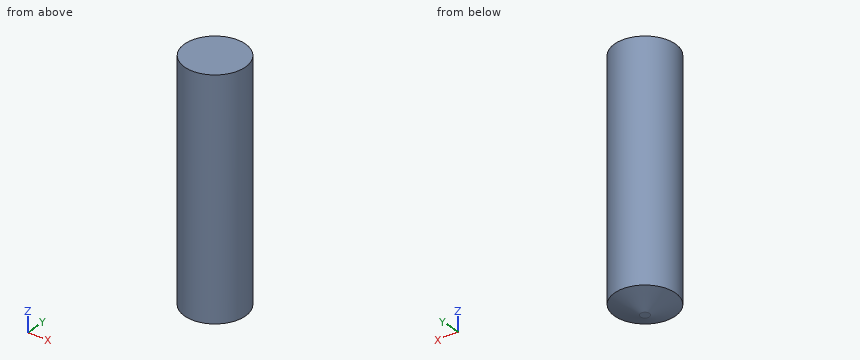
from build123d import *

# Parameters (mm, degrees)
CYLINDER_R     = 2.5
CYLINDER_DEPTH = 20


with BuildPart() as nozzle_revolution:
    # Sketch006 → Revolution (revolve)
    with BuildSketch(Plane.XZ):
        Polygon((-0.375, 0), (-2.5, 0.815711), (-2.5, 0), align=None)
    revolve(axis=Axis((0, 0, 0), (0, 0, 1)))


with BuildPart() as nozzle_cut:
    # Cylinder → Cylinder (new body)
    with BuildSketch(Plane.XY):
        Circle(CYLINDER_R)
    extrude(amount=CYLINDER_DEPTH)

    # Cut: cut nozzle-revolution
    add(nozzle_revolution.part, mode=Mode.SUBTRACT)


solid = nozzle_cut.part
Geometry: final body of the model. Coordinates: model frame, mm. Coordinates: 2 decimals unless noted, no trailing zeros. Loops run counter-clockwise (first coordinate to the right, second up) from the corner with the lowest first, then second, coordinate; pieces in that order, holes last. Notation, with made-up numbers: M 15.5,7 L 74.5,7 A26 ccw 74.5,33 Z; hole C 89,49 d8. An arc over 180 degrees is marked long. One line per item, written item: value. Start each with the question number.
1) Cut plane C-C (z = 13.5). Return loops of the section in (x, y), then the cut area to 3 significant figures.
2) Pin query (flat end, axial travel): P1, Ø3, axis at y = -2, z = 2.5, coming from the +X side; P2, Ø1, axis at x = -1.5, y = 1.5, coming from the -Z side; P3, Ø3, axis at x = 2, z = 4.5, coming from the +Y side; P4, Ø2, axis at y = 0.5, z = 8.5, coming from the -X side. Return the tip coordinate at first contact, or that it passes through.
3) Cut plane A-A (x = 0). Return loops of the section in (y, z) (3 decimals).
4) Material intervals for L1, parallel to X at y = -0.1, z = 5; L2, parallel to X at y = -2, z = 2.75; L3, parallel to Z at x = -1.7, y = -0.55, sorted ascending. Write a range as from..to.
Evaluation:
1. outline: C 0,0 d5
1. area: 19.6 mm^2
2. P1: x = 2.45
2. P2: z = 0.48
2. P3: y = 2.45
2. P4: x = -2.5
3. outline: M -2.5,0.816 L -0.375,0 L 0.375,0 L 2.5,0.816 L 2.5,20 L -2.5,20 Z
4. L1: -2.5..2.5
4. L2: -1.5..1.5
4. L3: 0.54..20
